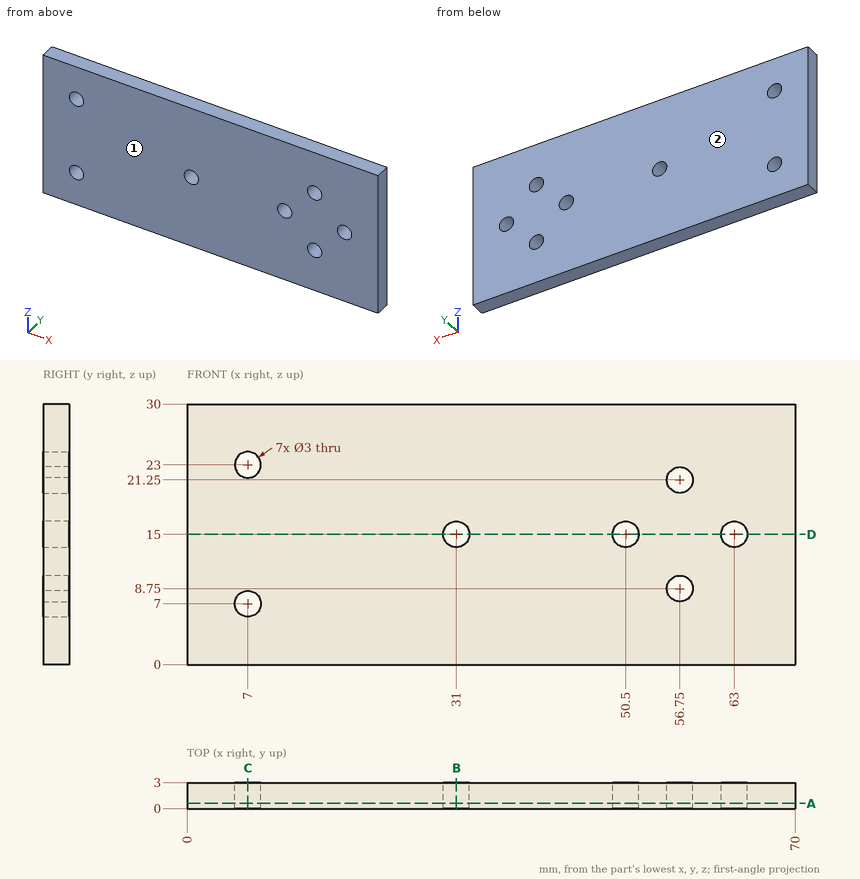
The figure shows three views and two pictorial views of one solid part (mm, origin at its lowest corner). Answer the questions. Coordinates: 2 decimals unless noted, no trailing zeros. Loops run counter-clockwise (first coordinate to the right, second up) from the corner with the lowest first, then second, coordinate; pieces in that order, holes last. Notation, with made-up numbers: (46, -4) - (97, -4) arc R17 ccw to (97, 26) - close; hole circle Ø3 at (23, -7.75). An arc over 180 degrees is marked (long way). Answer in a Markdown table with one row per item.
Q1. The mould has two halves that part along Y. Classify the marked faces 1 and 2: pulls with the +Y half, pulls with the -Y half, needs draft (parallel to the pull), parting line crosses it, or undercut.
Here are the results:
| item | result |
|---|---|
| face 1 | pulls with the -Y half |
| face 2 | pulls with the +Y half |
Q2. Find section D-D on z = 15. Write down the section's boundary in (x, y).
Here are the results:
| item | result |
|---|---|
| outline | (0, 0) - (29.5, 0) - (29.5, 3) - (0, 3) - close; (32.5, 0) - (49, 0) - (49, 3) - (32.5, 3) - close; (52, 0) - (61.5, 0) - (61.5, 3) - (52, 3) - close; (64.5, 0) - (70, 0) - (70, 3) - (64.5, 3) - close |
Q3. Given P1, Ø2.5, axis at x = 56.75, z = 21.25, coming from the +Y side, flat-ended and moving along its own axis, determine where the tip first touches the part or whether it passes through.
Here are the results:
| item | result |
|---|---|
| P1 | passes through |
Q4. Find section B-B on x = 31. Write down the section's boundary in (y, z).
Here are the results:
| item | result |
|---|---|
| outline | (0, 0) - (3, 0) - (3, 13.5) - (0, 13.5) - close; (0, 16.5) - (3, 16.5) - (3, 30) - (0, 30) - close |
Q5. Find section C-C on x = 7. Write down the section's boundary in (y, z), plus the area to 3 significant figures.
Here are the results:
| item | result |
|---|---|
| outline | (0, 0) - (3, 0) - (3, 5.5) - (0, 5.5) - close; (0, 8.5) - (3, 8.5) - (3, 21.5) - (0, 21.5) - close; (0, 24.5) - (3, 24.5) - (3, 30) - (0, 30) - close |
| area | 72.0 mm^2 |
Q6. Find section A-A on y = 0.6. Write down the section's boundary in (x, z), plus the area to 3 significant figures.
Here are the results:
| item | result |
|---|---|
| outline | (0, 0) - (70, 0) - (70, 30) - (0, 30) - close; hole circle Ø3 at (7, 7); hole circle Ø3 at (7, 23); hole circle Ø3 at (31, 15); hole circle Ø3 at (50.5, 15); hole circle Ø3 at (56.75, 8.75); hole circle Ø3 at (56.75, 21.25); hole circle Ø3 at (63, 15) |
| area | 2,050 mm^2 |
Q7. Straight lines are drawn through the part: line 1 along X through (y, z) = (1.25, 15); line 2 along X through (y, z) = (1.9, 22.5); line 3 along X through (y, z) = (1.8, 8.75). For each, find the intervals that lie inside material, in ascending order. Write a range as [from, to].
Here are the results:
| item | result |
|---|---|
| line 1 | x = [0, 29.5], [32.5, 49], [52, 61.5], [64.5, 70] |
| line 2 | x = [0, 5.59], [8.41, 55.92], [57.58, 70] |
| line 3 | x = [0, 55.25], [58.25, 70] |
